CAD build for the part. Positions are in the model's coordinates, mm. A direction names the side the tool comes from. Coordinates: 2 decimals unless noted, no trailing zeros. Loops run counter-clockwise (first coordinate to the right, second up) from the corner with the lowest first, then second, coordinate; pieces in that order, holes last. Notation, with made-up numbers: (25.5, -30) -> (30.5, -30) arc R26 ccw to (30.5, -11) -> close; hole circle Ø6 at (40.5, 71.25). An arc over 180 degrees is marked (long way). Answer as a JSON object with one key per item and string values. Group by question number.
from build123d import *

# Parameters (mm, degrees)
SKETCH1_R           = 8.9
SKETCH1_R_2         = 1.9
SKETCH1_R_3         = 1.4
SKETCH1_R_4         = 1.5
SKETCH1_W           = 20
SKETCH1_H           = 13
BOSS_EXTRUDE1_DEPTH = 3


with BuildPart() as part:
    # Sketch1 → Boss-Extrude1 (new body)
    with BuildSketch(Plane(origin=(0, 0, 0), x_dir=(1, 0, 0), z_dir=(0, 1, 0))):
        with BuildLine():
            Line((78.373949741, -14.153046231), (62.626050259, -12.971953769))
            ThreePointArc((62.626050259, -12.971953769), (59.334638578, -11.386710908), (58, -7.98595722))
            Line((58, -7.98595722), (58, 7.98595722))
            ThreePointArc((58, 7.98595722), (59.334638578, 11.386710908), (62.626050259, 12.971953769))
            Line((62.626050259, 12.971953769), (78.373949741, 14.153046231))
            ThreePointArc((78.373949741, 14.153046231), (81.665361422, 15.738289092), (83, 19.13904278))
            Line((83, 19.13904278), (83, 34.5))
            ThreePointArc((83, 34.5), (80.071067812, 41.571067812), (73, 44.5))
            Line((73, 44.5), (-89, 44.5))
            ThreePointArc((-89, 44.5), (-96.071067812, 41.571067812), (-99, 34.5))
            Line((-99, 34.5), (-99, 19.13904278))
            ThreePointArc((-99, 19.13904278), (-97.665361422, 15.738289092), (-94.373949741, 14.153046231))
            Line((-94.373949741, 14.153046231), (-43.626050259, 10.346953769))
            ThreePointArc((-43.626050259, 10.346953769), (-40.334638578, 8.761710908), (-39, 5.36095722))
            Line((-39, 5.36095722), (-39, -5.36095722))
            ThreePointArc((-39, -5.36095722), (-40.334638578, -8.761710908), (-43.626050259, -10.346953769))
            Line((-43.626050259, -10.346953769), (-94.373949741, -14.153046231))
            ThreePointArc((-94.373949741, -14.153046231), (-97.665361422, -15.738289092), (-99, -19.13904278))
            Line((-99, -19.13904278), (-99, -34.5))
            ThreePointArc((-99, -34.5), (-96.071067812, -41.571067812), (-89, -44.5))
            Line((-89, -44.5), (73, -44.5))
            ThreePointArc((73, -44.5), (80.071067812, -41.571067812), (83, -34.5))
            Line((83, -34.5), (83, -19.13904278))
            ThreePointArc((83, -19.13904278), (81.665361422, -15.738289092), (78.373949741, -14.153046231))
        make_face()
        Circle(SKETCH1_R, mode=Mode.SUBTRACT)
        with Locations((78, -18)):
            Circle(SKETCH1_R_2, mode=Mode.SUBTRACT)
        with Locations((77, -35)):
            Circle(SKETCH1_R_3, mode=Mode.SUBTRACT)
        with Locations((57, -35)):
            Circle(SKETCH1_R_3, mode=Mode.SUBTRACT)
        with Locations((49, -39.5)):
            Circle(SKETCH1_R_3, mode=Mode.SUBTRACT)
        with Locations((45, -16)):
            Circle(SKETCH1_R_3, mode=Mode.SUBTRACT)
        with Locations((22.273863607, -8.131727984)):
            Circle(SKETCH1_R_3, mode=Mode.SUBTRACT)
        with Locations((22.273863607, 8.131727984)):
            Circle(SKETCH1_R_3, mode=Mode.SUBTRACT)
        with Locations((10, -39.5)):
            Circle(SKETCH1_R_3, mode=Mode.SUBTRACT)
        with Locations((2, -35)):
            Circle(SKETCH1_R_3, mode=Mode.SUBTRACT)
        with Locations((8.131727984, -22.273863607)):
            Circle(SKETCH1_R_3, mode=Mode.SUBTRACT)
        with Locations((-8.131727984, -22.273863607)):
            Circle(SKETCH1_R_3, mode=Mode.SUBTRACT)
        with Locations((-18, -35)):
            Circle(SKETCH1_R_3, mode=Mode.SUBTRACT)
        with Locations((-26, -39.5)):
            Circle(SKETCH1_R_3, mode=Mode.SUBTRACT)
        with Locations((-22.273863607, -8.131727984)):
            Circle(SKETCH1_R_3, mode=Mode.SUBTRACT)
        with Locations((-22.273863607, 8.131727984)):
            Circle(SKETCH1_R_3, mode=Mode.SUBTRACT)
        with Locations((-8.131727984, 22.273863607)):
            Circle(SKETCH1_R_3, mode=Mode.SUBTRACT)
        with Locations((8.131727984, 22.273863607)):
            Circle(SKETCH1_R_3, mode=Mode.SUBTRACT)
        with Locations((45, 16)):
            Circle(SKETCH1_R_3, mode=Mode.SUBTRACT)
        with Locations((78, 18)):
            Circle(SKETCH1_R_2, mode=Mode.SUBTRACT)
        with Locations((77, 35)):
            Circle(SKETCH1_R_3, mode=Mode.SUBTRACT)
        with Locations((57, 35)):
            Circle(SKETCH1_R_3, mode=Mode.SUBTRACT)
        with Locations((49, 39.5)):
            Circle(SKETCH1_R_3, mode=Mode.SUBTRACT)
        with Locations((10, 39.5)):
            Circle(SKETCH1_R_3, mode=Mode.SUBTRACT)
        with Locations((2, 35)):
            Circle(SKETCH1_R_3, mode=Mode.SUBTRACT)
        with Locations((-18, 35)):
            Circle(SKETCH1_R_3, mode=Mode.SUBTRACT)
        with Locations((-26, 39.5)):
            Circle(SKETCH1_R_3, mode=Mode.SUBTRACT)
        with Locations((-60, 16)):
            Circle(SKETCH1_R_4, mode=Mode.SUBTRACT)
        with Locations((-60, -16)):
            Circle(SKETCH1_R_3, mode=Mode.SUBTRACT)
        with Locations((-65, -39.5)):
            Circle(SKETCH1_R_3, mode=Mode.SUBTRACT)
        with Locations((-73, -35)):
            Circle(SKETCH1_R_3, mode=Mode.SUBTRACT)
        with Locations((-93, -35)):
            Circle(SKETCH1_R_3, mode=Mode.SUBTRACT)
        with Locations((-94, -18)):
            Circle(SKETCH1_R_2, mode=Mode.SUBTRACT)
        with Locations((-94, 18.096449674)):
            Circle(SKETCH1_R_2, mode=Mode.SUBTRACT)
        with Locations((-93, 35)):
            Circle(SKETCH1_R_3, mode=Mode.SUBTRACT)
        with Locations((-73, 35)):
            Circle(SKETCH1_R_3, mode=Mode.SUBTRACT)
        with Locations((-65, 39.5)):
            Circle(SKETCH1_R_3, mode=Mode.SUBTRACT)
        with BuildLine():
            Line((-33, 20), (-58, 20))
            ThreePointArc((-58, 20), (-59.414213562, 20.585786438), (-60, 22))
            Line((-60, 22), (-60, 36.5))
            ThreePointArc((-60, 36.5), (-59.414213562, 37.914213562), (-58, 38.5))
            Line((-58, 38.5), (-33, 38.5))
            ThreePointArc((-33, 38.5), (-31.585786438, 37.914213562), (-31, 36.5))
            Line((-31, 36.5), (-31, 22))
            ThreePointArc((-31, 22), (-31.585786438, 20.585786438), (-33, 20))
        make_face(mode=Mode.SUBTRACT)
        with Locations((35.205, 0)):
            Rectangle(SKETCH1_W, SKETCH1_H, mode=Mode.SUBTRACT)
        with BuildLine():
            Line((45.5, 36.5), (45.5, 22))
            ThreePointArc((45.5, 22), (44.914213562, 20.585786438), (43.5, 20))
            Line((43.5, 20), (17, 20))
            ThreePointArc((17, 20), (15.585786438, 20.585786438), (15, 22))
            Line((15, 22), (15, 36.5))
            ThreePointArc((15, 36.5), (15.585786438, 37.914213562), (17, 38.5))
            Line((17, 38.5), (43.5, 38.5))
            ThreePointArc((43.5, 38.5), (44.914213562, 37.914213562), (45.5, 36.5))
        make_face(mode=Mode.SUBTRACT)
        with BuildLine():
            Line((43.5, -38.5), (17, -38.5))
            ThreePointArc((17, -38.5), (15.585786438, -37.914213562), (15, -36.5))
            Line((15, -36.5), (15, -22))
            ThreePointArc((15, -22), (15.585786438, -20.585786438), (17, -20))
            Line((17, -20), (43.5, -20))
            ThreePointArc((43.5, -20), (44.914213562, -20.585786438), (45.5, -22))
            Line((45.5, -22), (45.5, -36.5))
            ThreePointArc((45.5, -36.5), (44.914213562, -37.914213562), (43.5, -38.5))
        make_face(mode=Mode.SUBTRACT)
        with BuildLine():
            Line((-31, -22), (-31, -36.5))
            ThreePointArc((-31, -36.5), (-31.585786438, -37.914213562), (-33, -38.5))
            Line((-33, -38.5), (-58, -38.5))
            ThreePointArc((-58, -38.5), (-59.414213562, -37.914213562), (-60, -36.5))
            Line((-60, -36.5), (-60, -22))
            ThreePointArc((-60, -22), (-59.414213562, -20.585786438), (-58, -20))
            Line((-58, -20), (-33, -20))
            ThreePointArc((-33, -20), (-31.585786438, -20.585786438), (-31, -22))
        make_face(mode=Mode.SUBTRACT)
    extrude(amount=BOSS_EXTRUDE1_DEPTH)


solid = part.part
Item 1: Band-saw the part on C-C, the plane x = 36.5. List the corners of the cut face in (y, z).
Item 2: 3-axis set-ups, long thin cutter, end or side, ignore diameter. For faces 1 (the cylindrical face through (59.3, 1.48, -11.35)), 2 (the flat face through (-69.355, 1.479, -12.277)), 3 (the cylindrical face through (-1.93, 1.48, 8.69)): which of +Z, -Z, +X, -X, +Y, -Y reach the whole face in a straight line?
Item 3: Band-saw the part on B-B, the plane z = 0. List the corners of the cut face in (x, y) (3 decimals), and give its area (3 significant figures).
Item 4: Pull direction Z, two halves, no side cores. Call faces 4 (the cylindrical face through (-95.99, 1.48, -41.65)), 5 (the cylindrical face through (-97.701, 1.479, -15.777)), 6 (the cylindrical face through (81.701, 1.479, 15.777)), 7 (the flat face through (-9, 3, -1)): +Z half, -Z half, draft (parallel to the pull), parting line (faces both ways), or undercut.
Item 5: Flat gauge pins, fed straight in: P1, Ø1.7, axis at x = 2, z = 35, coming from the -Y side; P2, Ø1.5, axis at y = 2, z = 0.5, coming from the -X side. Where does each tip first touch, or does it go through?
Item 6: Band-saw the part on A-A, the plane x = -83. List the corners of the cut face in (y, z).
Item 7: Band-saw the part on D-D, the plane y = 1.6. Count the separate pieces of the cut face and the enclosed holes in it, and give its area (3 significant figures).
Item 8: Drill centre lines: L1, parallel to Z at x = 19, y = 0.95; L2, parallel to X at y = 1.4, z = -4 (3 decimals); L3, parallel to X at y = 2.7, z = -26.5. Where is each one in solid material? Low to high.
Reply:
{
 "1": {"outline": "(0, -44.5) -> (3, -44.5) -> (3, -38.5) -> (0, -38.5) -> close; (0, -20) -> (3, -20) -> (3, -6.5) -> (0, -6.5) -> close; (0, 6.5) -> (3, 6.5) -> (3, 20) -> (0, 20) -> close; (0, 38.5) -> (3, 38.5) -> (3, 44.5) -> (0, 44.5) -> close"},
 "2": {"face 1": "+X, +Y, -Y", "face 2": "-X, +Y, -Y", "face 3": "+Y, -Y"},
 "3": {"outline": "(-39, 0) -> (-8.9, 0) -> (-8.9, 3) -> (-39, 3) -> close; (8.9, 0) -> (25.205, 0) -> (25.205, 3) -> (8.9, 3) -> close; (45.205, 0) -> (58, 0) -> (58, 3) -> (45.205, 3) -> close", "area": "178 mm²"},
 "4": {"face 4": "-Z half", "face 5": "undercut", "face 6": "undercut", "face 7": "draft"},
 "5": {"P1": "through", "P2": "x = -39"},
 "6": {"outline": "(0, -44.5) -> (3, -44.5) -> (3, -13.3) -> (0, -13.3) -> close; (0, 13.3) -> (3, 13.3) -> (3, 44.5) -> (0, 44.5) -> close"},
 "7": {"separate pieces": "1", "enclosed holes": "42", "area": "11,000 mm²"},
 "8": {"L1": "-44.5 to -38.5, -20 to 20, 38.5 to 44.5", "L2": "-39 to -7.95, 7.95 to 25.205, 45.205 to 58", "L3": "-99 to -60, -31 to 15, 45.5 to 83"}
}
